Can you work these out from the drawing? Everything is in mm from the part's minimum corner. Give positions to 0.01 mm unless a question says otherwise; leave off trailing zeros. Write each loop counter-clockwise with the first axis right and the second up, starting at its lowest first coordinate (ties: lowest second). Pieces come first, ordered by that corner, then holes. Notation, with made-up numbers: (-24, 19.5) - (2, 19.5) arc R8 cw to (2, 34.5) - close; hole circle Ø6 at (-21.75, 49.5). An arc over 180 degrees is marked (long way). Use a Markdown table: item, result. Add a question column.
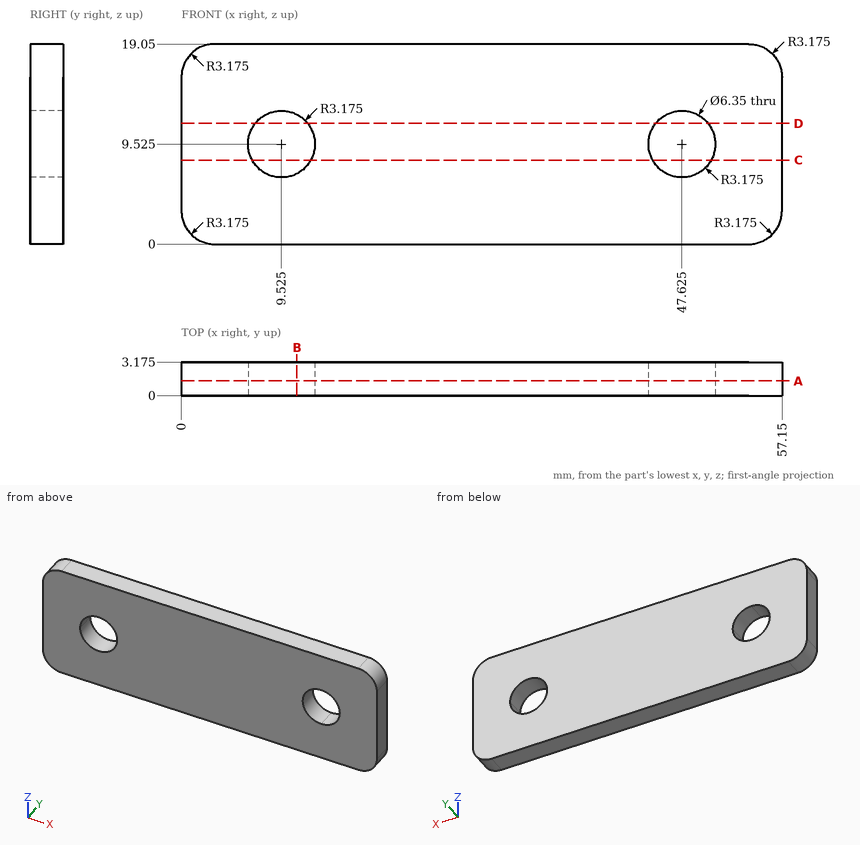
Q1. Suppose I cut it at A-A (y = 1.4). Please give me the cut outline in (x, z) (3 decimals).
Q2. Suppose I cut it at C-C (z = 8). Please give me the cut outline in (x, y) (3 decimals).
Q3. Suppose I cut it at B-B (x = 11). Please give me the cut outline in (y, z) (3 decimals).
Q4. If I drill on probe 1 along X at (y, z) = (2.1, 11.75); probe 2 along X at (y, z) = (0.3, 7); probe 3 along Z at (x, y) = (45.5, 1.45), over which ranges is the centre line in solid material (lowest first)? Write a range as [from, to].
Q5. Suppose I cut it at D-D (z = 11.5). Please give me the cut outline in (x, y) (3 decimals), and give its area (3 significant figures).
Q6. I'm going to push flat-ended pins straight in: P1, Ø1, axis at y = 1, z = 2, coming from the -X side; P2, Ø5, axis at x = 47.625, z = 9.525, coming from the -Y side. Where does each tip first touch, or does it pass through?
Derived:
| question | item | result |
|---|---|---|
| 1 | outline | (0, 3.175) arc R3.175 ccw to (3.175, 0) - (53.975, 0) arc R3.175 ccw to (57.15, 3.175) - (57.15, 15.875) arc R3.175 ccw to (53.975, 19.05) - (3.175, 19.05) arc R3.175 ccw to (0, 15.875) - close; hole (6.35, 9.525) arc R3.175 ccw (long way) to (9.525, 12.7) arc R3.175 ccw to start; hole (47.625, 6.35) arc R3.175 ccw to (50.8, 9.525) arc R3.175 ccw (long way) to start |
| 2 | outline | (0, 0) - (6.74, 0) - (6.74, 3.175) - (0, 3.175) - close; (12.31, 0) - (44.84, 0) - (44.84, 3.175) - (12.31, 3.175) - close; (50.41, 0) - (57.15, 0) - (57.15, 3.175) - (50.41, 3.175) - close |
| 3 | outline | (0, 0) - (3.175, 0) - (3.175, 6.713) - (0, 6.713) - close; (0, 12.337) - (3.175, 12.337) - (3.175, 19.05) - (0, 19.05) - close |
| 4 | probe 1 | [0, 7.26], [11.79, 45.36], [49.89, 57.15] |
| 4 | probe 2 | [0, 7.6], [11.45, 45.7], [49.55, 57.15] |
| 4 | probe 3 | [0, 7.17], [11.88, 19.05] |
| 5 | outline | (0, 0) - (7.039, 0) - (7.039, 3.175) - (0, 3.175) - close; (12.011, 0) - (45.139, 0) - (45.139, 3.175) - (12.011, 3.175) - close; (50.111, 0) - (57.15, 0) - (57.15, 3.175) - (50.111, 3.175) - close |
| 5 | area | 150 mm² |
| 6 | P1 | x = 0.07 |
| 6 | P2 | through |
